```python
from build123d import *

# Parameters (mm, degrees)
F0_R     = 21.720665
F0_R_2   = 16.520494
F1_DEPTH = 31.75
F0_W     = 84.640459
F0_H     = 65.472521
F2_DEPTH = 12.7
F3_W     = 86.387612
F3_H     = 35.076849
F4_DEPTH = 31.75
F5_R     = 3.429
F6_DEPTH = 25.4


with BuildPart() as f1:
    # F0 (on Front) → F1 (new body, symmetric)
    with BuildSketch(Plane.XZ):
        Circle(F0_R)
        Circle(F0_R_2, mode=Mode.SUBTRACT)
    extrude(amount=F1_DEPTH, both=True)

    # F0 (on Front) → F2 (join, symmetric)
    with BuildSketch(Plane.XZ):
        with Locations((1.507592, -0.216593)):
            Rectangle(F0_W, F0_H)
        Circle(F0_R, mode=Mode.SUBTRACT)
    extrude(amount=F2_DEPTH, both=True)

    # F3 (on Front) → F4 (cut, symmetric)
    with BuildSketch(Plane.XZ):
        with Locations((2.319131, 17.538424)):
            Rectangle(F3_W, F3_H)
    extrude(amount=F4_DEPTH, both=True, mode=Mode.SUBTRACT)

    # F5 (on face) → F6 (cut)
    with BuildSketch(Plane.XY):
        with Locations((-30.424622, 0)):
            Circle(F5_R)
        with Locations((31.681519, 0)):
            Circle(F5_R)
    extrude(amount=-F6_DEPTH, mode=Mode.SUBTRACT)


solid = f1.part
```
Geometry check sheet. Reference: the model listing, model coordinates, mm. A direction names the side the tool comes from. Coordinates: 2 decimals unless noted, no trailing zeros. Write each loop counter-clockwise with the first axis right and the second up, starting at its lowest first coordinate (ties: lowest second). Pieces come first, ordered by that corner, then holes. Notation, with made-up numbers: M 8.25,79 L 44.25,79 A34 ccw 44.25,115 Z; hole C 28.5,-22 d9. An arc over 180 degrees is marked long. Answer as a JSON object with one key per item and string values.
1. Draft check along X on faces 5 (the cylindrical face through (-0.478, -22.358, -21.715)), 6 (the cylindrical face through (34.85, -1.31, -12.52)), 7 (the flat face through (1, 12.7, -24)). Enter one of: released by +X, released by -X, zero draft, split by the parting line, or undercut.
Answers below:
{"face 5": "split by the parting line", "face 6": "undercut", "face 7": "zero draft"}
2. Go/stop test with flat-tipped pins: pin 1 Ø1 at (x, y) = (10.5, -13.5) entering from -Z; pin 2 Ø4 at (y, z) = (-15, -17.5) entering from +X; pin 3 Ø2 at (x, y) = (31, 1.5) entering from +Z. Record where each tip stops, or that it passes through.
Answers below:
{"pin 1": "stops at z = -19.28", "pin 2": "stops at x = 15.22", "pin 3": "stops at z = -25.4"}
3. Tool access check on faces 1 (the flat face through (2, -31.75, -17)), 2 (the flat face through (1, -12.7, -24)), 3 (the cylindrical face through (-27.154, 1.03, -12.522)), 4 (the cylindrical face through (-0.478, 22.092, -21.715)). Record the directions out of +Z, -Z, +X, -X, +Y, -Y that give a thin tool (end or side, any length) a straight path to the whole face; none if there is none.
Answers below:
{"face 1": "+Z, -Z, +X, -X, -Y", "face 2": "-Z, -Y", "face 3": "+Z", "face 4": "-Z, +Y"}
4. Section check B-B, the plane x = 0. Enter the section's corners in (y, z).
Answers below:
{"outline": "M -31.75,-21.72 L -12.7,-21.72 L -12.7,-32.95 L 12.7,-32.95 L 12.7,-21.72 L 31.75,-21.72 L 31.75,-16.52 L -31.75,-16.52 Z"}
5. Section check C-C, the plane y = 0. Enter the section's corners in (x, z).
Answers below:
{"outline": "M -40.81,-32.95 L 43.83,-32.95 L 43.83,0 L 35.11,0 L 35.11,-25.4 L 28.25,-25.4 L 28.25,0 L 16.52,0 A16.52 cw -16.52,0 L -27,0 L -27,-25.4 L -33.85,-25.4 L -33.85,0 L -40.81,0 Z"}
6. Section check D-D, the plane z = -28. Enter the section's corners in (x, y).
Answers below:
{"outline": "M -40.81,-12.7 L 43.83,-12.7 L 43.83,12.7 L -40.81,12.7 Z"}
7. Scan lines: L1, parallel to X at y = -9.5, z = -11; L2, parallel to Y at x = 22, z = -14; L3, parallel to X at y = -10.5, z = -12. Record each from-to range of solid material in increasing order.
Answers below:
{"L1": "x = -40.81 to -12.33, 12.33 to 43.83", "L2": "y = -12.7 to 12.7", "L3": "x = -40.81 to -11.35, 11.35 to 43.83"}
8. Section check A-A, the plane z = -24. Enter the section's corners in (x, y).
Answers below:
{"outline": "M -40.81,-12.7 L 43.83,-12.7 L 43.83,12.7 L -40.81,12.7 Z; hole C -30.42,0 d6.86; hole C 31.68,0 d6.86"}
